```python
from build123d import *

# Parameters (mm, degrees)
SKETCH1_W               = 29.85
SKETCH1_H               = 30
BOSS_EXTRUDE1_DEPTH     = 12.5
SKETCH2_W               = 5
SKETCH2_H               = 20
CUT_EXTRUDE1_DEPTH      = 45.127910669
CUT_EXTRUDE3_DEPTH      = 45.127910669
CUT_EXTRUDE5_DEPTH      = 45.127910669
SKETCH8_W               = 6.842575397
SKETCH8_H               = 30
BOSS_EXTRUDE5_DEPTH     = 3.65
SKETCH9_W               = 6.842575397
SKETCH9_H               = 30
BOSS_EXTRUDE6_DEPTH     = 3.65
CUT_EXTRUDE7_DEPTH      = 47.674404212
CUT_EXTRUDE7_DEPTH_BACK = 47.674404212
SKETCH4_R               = 1.5
FILLET17_R              = 0.25
FILLET19_R              = 0.25


with BuildPart() as part:
    # Sketch1 → Boss-Extrude1 (new body)
    with BuildSketch(Plane.XY):
        with Locations((14.925, 15)):
            Rectangle(SKETCH1_W, SKETCH1_H)
    extrude(amount=BOSS_EXTRUDE1_DEPTH)

    # Sketch2 → Cut-Extrude1 (cut, through all)
    with BuildSketch(Plane.XY.offset(12.5)):
        with Locations((14.925, 15)):
            Rectangle(SKETCH2_W, SKETCH2_H)
    extrude(amount=-CUT_EXTRUDE1_DEPTH, mode=Mode.SUBTRACT)

    # Sketch5 → Cut-Extrude3 (cut, through all)
    with BuildSketch(Plane.XZ):
        with BuildLine():
            Line((0, 6.842575397), (-5.709638119, 18.35105476))
            Line((-5.709638119, 18.35105476), (14.925, 23.822049063))
            Line((14.925, 23.822049063), (34.386752026, 18.35105476))
            Line((34.386752026, 18.35105476), (29.85, 6.842575397))
            ThreePointArc((29.85, 6.842575397), (14.925, 12.5), (0, 6.842575397))
        make_face()
    extrude(amount=-CUT_EXTRUDE3_DEPTH, mode=Mode.SUBTRACT)

    # Sketch7 → Cut-Extrude5 (cut, through all)
    with BuildSketch(Plane(origin=(29.85, 0, 0), x_dir=(0, 0, -1), z_dir=(1, 0, 0))):
        with BuildLine():
            Line((-6.842575397, 0), (-6.842575397, -1.983675783))
            Line((-6.842575397, -1.983675783), (-14.601311023, -1.983675783))
            Line((-14.601311023, -1.983675783), (-14.601311023, 5))
            Line((-14.601311023, 5), (-12.360777707, 5))
            add(Edge.make_bspline(
                [(-6.842575397, 0), (-11.686120983, 0.298823628), (-12.360777707, 5)],
                knots=[0, 0, 0, 1, 1, 1], degree=2))
        make_face()
    extrude(amount=-CUT_EXTRUDE5_DEPTH, mode=Mode.SUBTRACT)

    # Sketch8 → Boss-Extrude5 (add)
    with BuildSketch(Plane(origin=(29.85, 0, 0), x_dir=(0, 0, -1), z_dir=(1, 0, 0))):
        with Locations((-3.421287699, 15)):
            Rectangle(SKETCH8_W, SKETCH8_H)
    extrude(amount=BOSS_EXTRUDE5_DEPTH)

    # Sketch9 → Boss-Extrude6 (add)
    with BuildSketch(Plane.ZY):
        with Locations((3.421287699, 15)):
            Rectangle(SKETCH9_W, SKETCH9_H)
    extrude(amount=BOSS_EXTRUDE6_DEPTH)

    # Sketch4 → Cut-Extrude7 (cut, two sides: drawn at the far end of the back side and taken through both)
    with BuildSketch(Plane(origin=(29.85, 0, 0), x_dir=(0, 0, -1), z_dir=(1, 0, 0)).offset(-CUT_EXTRUDE7_DEPTH_BACK)):
        with Locations((-3.5, 25)):
            Circle(SKETCH4_R)
        with Locations((-3.5, 5)):
            Circle(SKETCH4_R)
    extrude(amount=CUT_EXTRUDE7_DEPTH + CUT_EXTRUDE7_DEPTH_BACK, mode=Mode.SUBTRACT)

    # Fillet17
    fillet17_edges = [part.edges().sort_by_distance(p)[0] for p in [
        (-3.65, 25, 5),
        (33.5, 25, 5),
        (-3.65, 5, 5),
        (33.5, 5, 5),
    ]]
    fillet(fillet17_edges, radius=FILLET17_R)

    # Fillet19
    # the kernel refuses this fillet: 0.25 mm, written as the material it takes off along each edge
    with BuildSketch(Plane(origin=(17.425, 25, 12.360777707), x_dir=(0.9930996963041147, 0, -0.11727315635163624), z_dir=(0, -1, 0))) as fillet19_piece_1:
        with BuildLine():
            CenterArc((0.28125848, -0.249995069), FILLET19_R, 89.640140573, 97.094614091)
            Line((0.032983556, -0.279313358), (0, 0))
            ThreePointArc((0, 0), (0.141414326, 0.000444094), (0.282828652, 0))
        make_face()
    extrude(amount=20, mode=Mode.SUBTRACT)
    with BuildSketch(Plane(origin=(14.925, 25, -10.015728977), x_dir=(-0.13857412950442824, 0, 0.9903520639813349), z_dir=(-0.9903520639813349, 0, -0.13857412950442824))) as fillet19_piece_2_section:
        with BuildLine():
            CenterArc((22.515728977 - FILLET19_R, FILLET19_R), FILLET19_R, 270, 90)
            Line((22.515728977 - FILLET19_R, 0), (22.515728977, 0))
            Line((22.515728977, 0), (22.515728977, FILLET19_R))
        make_face()
    fillet19_piece_2 = revolve(axis=Axis((14.925, 25, -10.015728977), (0, 1, 0)), revolution_arc=15.930691333, mode=Mode.PRIVATE)
    fillet19_piece_2 = split(fillet19_piece_2, bisect_by=Plane(origin=(12.425, 25.070178335, 12.429821665), z_dir=(1, 0, 0)), keep=Keep.TOP, mode=Mode.PRIVATE)
    fillet19_piece_2 = split(fillet19_piece_2, bisect_by=Plane(origin=(17.425, 25.070178335, 12.429821665), z_dir=(-1, 0, 0)), keep=Keep.TOP, mode=Mode.PRIVATE)
    add(fillet19_piece_2, mode=Mode.SUBTRACT)
    with BuildSketch(Plane(origin=(14.925, 30, -10.015728977), x_dir=(0.6834024940823613, 0, 0.7300418009141724), z_dir=(0.7300418009141724, 0, -0.6834024940823613))) as fillet19_piece_3_section:
        with BuildLine():
            CenterArc((22.515728977 - FILLET19_R, FILLET19_R), FILLET19_R, 270, 90)
            Line((22.515728977, FILLET19_R), (22.515728977, 0))
            Line((22.515728977, 0), (22.515728977 - FILLET19_R, 0))
        make_face()
    fillet19_piece_3 = revolve(axis=Axis((14.925, 30, -10.015728977), (0, -1, 0)), revolution_arc=86.220203027, mode=Mode.PRIVATE)
    fillet19_piece_3 = split(fillet19_piece_3, bisect_by=Plane(origin=(14.925, 29.93245071, 6.842575397), z_dir=(0, 0, 1)), keep=Keep.TOP, mode=Mode.PRIVATE)
    add(fillet19_piece_3, mode=Mode.SUBTRACT)
    with BuildSketch(Plane(origin=(12.425, 25, 12.360777707), x_dir=(-0.9930996963041147, 0, -0.1172731563516355), z_dir=(0, -1, 0))) as fillet19_piece_4:
        with BuildLine():
            CenterArc((0.28125848, 0.249995069), FILLET19_R, 173.265245336, 97.094614091)
            Line((0.032983556, 0.279313358), (0, 0))
            ThreePointArc((0, 0), (0.141414326, -0.000444094), (0.282828652, 0))
        make_face()
    extrude(amount=20, mode=Mode.SUBTRACT)
    with BuildSketch(Plane(origin=(17.425, 25.707071631, 12.360777707), x_dir=(0.9930996963041131, 0, -0.11727315635164862), z_dir=(0, -1, 0))) as fillet19_piece_5a_section:
        with BuildLine():
            CenterArc((0.28125848, -0.249995069), FILLET19_R, 89.640140573, 97.094614091)
            Line((0.032983556, -0.279313358), (0, 0))
            ThreePointArc((0, 0), (0.141414326, 0.000444094), (0.282828652, 0))
        make_face()
    fillet19_piece_5a = extrude(amount=20.707071631, mode=Mode.PRIVATE)
    fillet19_piece_5a = split(fillet19_piece_5a, bisect_by=Plane(origin=(17.489598012, 25, 12.288810309), z_dir=(0, 1, 0)), keep=Keep.TOP, mode=Mode.PRIVATE)
    with BuildSketch(Plane(origin=(14.925, 25, -10.015728977), x_dir=(-0.13857412950442824, 0, 0.9903520639813349), z_dir=(-0.9903520639813349, 0, -0.13857412950442824))) as fillet19_piece_5b_section:
        with BuildLine():
            CenterArc((22.515728977 - FILLET19_R, FILLET19_R), FILLET19_R, 270, 90)
            Line((22.515728977 - FILLET19_R, 0), (22.515728977, 0))
            Line((22.515728977, 0), (22.515728977, FILLET19_R))
        make_face()
    fillet19_piece_5b = revolve(axis=Axis((14.925, 25, -10.015728977), (0, 1, 0)), revolution_arc=15.930691333, mode=Mode.PRIVATE)
    fillet19_piece_5b = split(fillet19_piece_5b, bisect_by=Plane(origin=(17.425, 25.056986655, 12.26732893), z_dir=(1, 0, 0)), keep=Keep.TOP, mode=Mode.PRIVATE)
    fillet19_piece_5 = fillet19_piece_5a & fillet19_piece_5b
    add(fillet19_piece_5, mode=Mode.SUBTRACT)
    with BuildSketch(Plane(origin=(14.925, 25, -10.015728977), x_dir=(-0.13857412950442824, 0, 0.9903520639813349), z_dir=(-0.9903520639813349, 0, -0.13857412950442824))) as fillet19_piece_6a_section:
        with BuildLine():
            CenterArc((22.515728977 - FILLET19_R, FILLET19_R), FILLET19_R, 270, 90)
            Line((22.515728977 - FILLET19_R, 0), (22.515728977, 0))
            Line((22.515728977, 0), (22.515728977, FILLET19_R))
        make_face()
    fillet19_piece_6a = revolve(axis=Axis((14.925, 25, -10.015728977), (0, 1, 0)), revolution_arc=15.930691333, mode=Mode.PRIVATE)
    fillet19_piece_6a = split(fillet19_piece_6a, bisect_by=Plane(origin=(12.425, 25.056986602, 12.267328652), z_dir=(-1, 0, 0)), keep=Keep.TOP, mode=Mode.PRIVATE)
    with BuildSketch(Plane(origin=(12.425, 25.707071631, 12.360777707), x_dir=(-0.9930996963041131, 0, -0.11727315635164788), z_dir=(0, -1, 0))) as fillet19_piece_6b_section:
        with BuildLine():
            CenterArc((0.28125848, 0.249995069), FILLET19_R, 173.265245336, 97.094614091)
            Line((0.032983556, 0.279313358), (0, 0))
            ThreePointArc((0, 0), (0.141414326, -0.000444094), (0.282828652, 0))
        make_face()
    fillet19_piece_6b = extrude(amount=20.707071631, mode=Mode.PRIVATE)
    fillet19_piece_6b = split(fillet19_piece_6b, bisect_by=Plane(origin=(12.360401988, 25, 12.288810309), z_dir=(0, 1, 0)), keep=Keep.TOP, mode=Mode.PRIVATE)
    fillet19_piece_6 = fillet19_piece_6a & fillet19_piece_6b
    add(fillet19_piece_6, mode=Mode.SUBTRACT)


solid = part.part
```
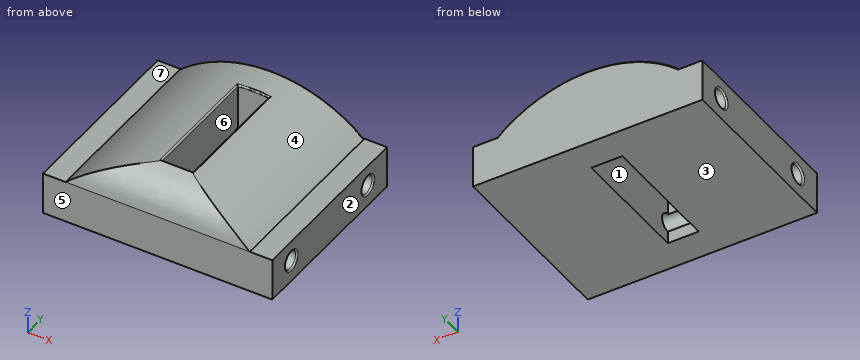
The listing builds one solid part. Answer for the finished solid, in the listing's coordinates (mm). Face numbers are marked on the shaded views. A direction names the side the tool comes from. Round coordinates to 2 decimals unless told otherwise and drop trailing zeros. Write each loop counter-clockwise with the first axis right and the second up, starting at its lowest first coordinate (ties: lowest second). Pieces come first, ordered by that corner, then holes. Notation, with made-up numbers: (86.5, 47.5) -> (109.5, 47.5) arc R12 ccw to (109.5, 53.5) -> close; hole circle Ø2 at (-6.5, -11). An arc over 180 degrees is marked (long way). Use CSV: the item, a comma, the result in double quotes. Start each with the question number.
(1) Which of the six approach directions +Z, -Z, +X, -X, +Y, -Y give full straight-line access (tool end or side, diameter ignored) to the marked faces 5, 6 and 7?
(2) The mould has two halves that part along X. Classify the marked faces 1, 2, 3 and 4: released by +X, released by -X, zero draft, split by the parting line, or undercut.
(3) Section C-C on y = 8.5 is taken. Give the vertices of the cut face in (x, z) (3 decimals), then the cut area to 3 significant figures.
(4) Section D-D on x = 28 is taken. Count the separate pieces of the cut face and the enclosed holes in it, then the cut area to 3 significant figures.
(5) Each of these flat-tipped pins is pushed along its axis until it touches: pin 1 (2 mm diameter, centred on x = -1.5, y = 10.5, fed in from +Z); pin 2 (4 mm diameter, centred on x = 15.5, z = 9, fed in from -Y). Where does it stop, or does it pass through?
(6) Consider L1, parallel to Y at x = 8, z = 3.5; L2, parallel to X at y = 9.5, z = 2 (3 decimals); L3, parallel to Y at x = 14.5, z = 3.5. Determine where each line is inside the solid, lowest interval first. Write a range as from..to.
(7) Section A-A on z = 6 is taken. Give the vertices of the cut face in (x, y) (3 decimals).
(8) Section B-B on z = 3.5 is taken. Give the vertices of the cut face in (x, y) (3 decimals).
A:
1,face 5,"+Z, -Z, +X, -X, -Y"
1,face 6,"+Z, -Z"
1,face 7,"+Z, -X, +Y, -Y"
2,face 1,"undercut"
2,face 2,"released by +X"
2,face 3,"zero draft"
2,face 4,"split by the parting line"
3,outline,"(-3.65, 0) -> (12.425, 0) -> (12.425, 12.08) arc R0.25 ccw to (12.144, 12.328) arc R22.516 ccw to (0, 6.843) -> (-3.65, 6.843) -> close; (17.425, 0) -> (33.5, 0) -> (33.5, 6.843) -> (29.85, 6.843) arc R22.516 ccw to (17.706, 12.328) arc R0.25 ccw to (17.425, 12.08) -> close"
3,area,"308 mm²"
4,separate pieces,"1"
4,enclosed holes,"2"
4,area,"235 mm²"
5,pin 1,"stops at z = 6.84"
5,pin 2,"stops at y = 0.01"
6,L1,"y = 0..3.5, 6.5..23.5, 26.5..30"
6,L2,"x = -3.65..12.425, 17.425..33.5"
6,L3,"y = 0..3.5, 26.5..30"
7,outline,"(-3.65, 0) -> (33.5, 0) -> (33.5, 30) -> (-3.65, 30) -> close; hole (12.425, 5) -> (17.425, 5) -> (17.425, 25) -> (12.425, 25) -> close"
8,outline,"(-3.65, 0) -> (33.5, 0) -> (33.5, 3.25) arc R0.25 ccw to (33.25, 3.5) -> (-3.4, 3.5) arc R0.25 ccw to (-3.65, 3.25) -> close; (-3.65, 6.75) arc R0.25 ccw to (-3.4, 6.5) -> (12.425, 6.5) -> (12.425, 23.5) -> (-3.4, 23.5) arc R0.25 ccw to (-3.65, 23.25) -> close; (-3.65, 26.75) arc R0.25 ccw to (-3.4, 26.5) -> (33.25, 26.5) arc R0.25 ccw to (33.5, 26.75) -> (33.5, 30) -> (-3.65, 30) -> close; (17.425, 6.5) -> (33.25, 6.5) arc R0.25 ccw to (33.5, 6.75) -> (33.5, 23.25) arc R0.25 ccw to (33.25, 23.5) -> (17.425, 23.5) -> close"
